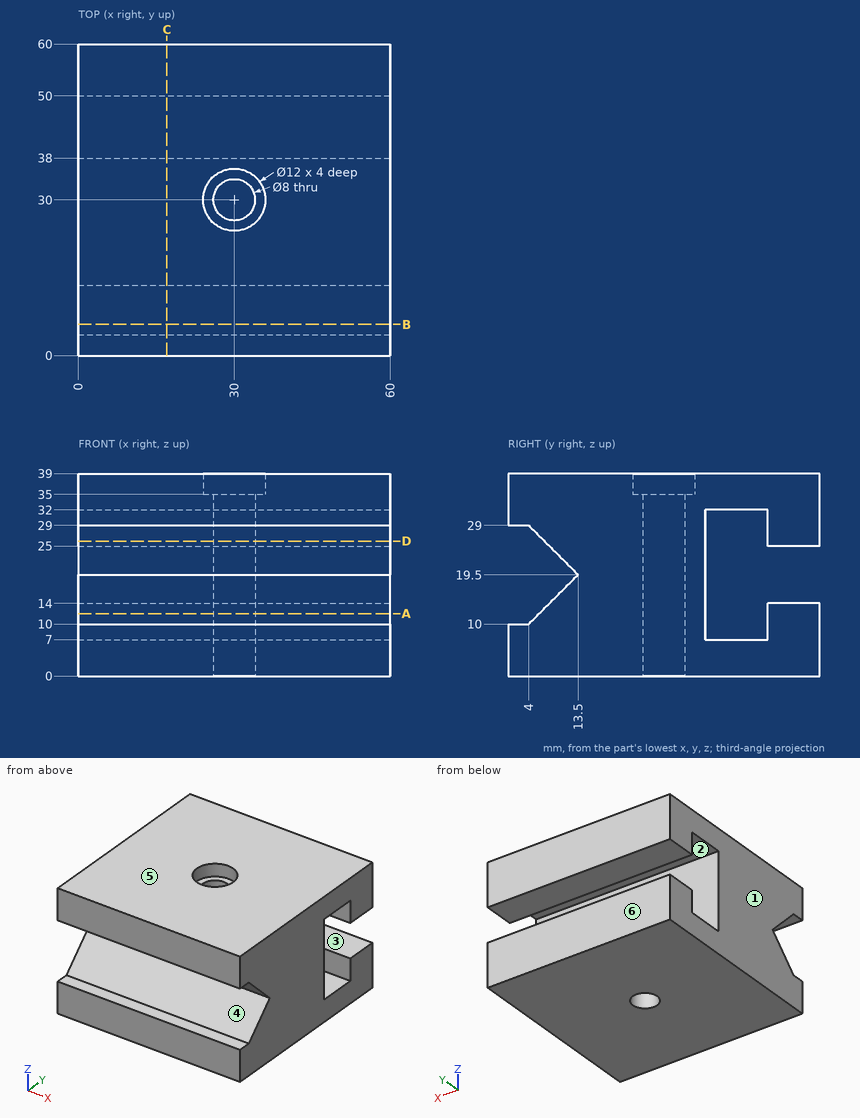
The figure shows three views and two pictorial views of one solid part (mm, origin at its lowest corner). Answer the questions. A direction names the side the tool comes from. Give positions to 0.01 mm unless a question says otherwise; leave off trailing zeros. Loops run counter-clockwise (first coordinate to the right, second up) from the corner with the lowest first, then second, coordinate; pieces in that order, holes last. Notation, with made-up numbers: (8.25, -25.5) -> (58.25, -25.5) arc R20 cw to (58.25, -21.5) -> close; hole circle Ø7 at (62.25, 44.5). An arc over 180 degrees is marked (long way). Use a Markdown table: item, result. Add a question column.
1. A flat-ended cylindrical pin translates along its axis: pin 1 Ø3.5 at (x, y) = (32.5, 27.5) entering from +Z. Find the tip coordinate at first contact, or state that the pin passes through.
2. Determine the mould class of the marked faces 4, 5 and 6 for opening direction Z: released by +Z, released by -Z, zero draft, split by the parting line, or undercut.
3. Find the intervals of material crossed by probe 1 along X at (y, z) = (30, 19); probe 2 along X at (y, z) = (30, 37.6); probe 3 along Z at (x, y) = (17, 55.5), in increasing order.
4. Section D-D on z = 26 is taken. Determine the outline of the cut face in (x, y).
5. For the marked faces 1, 2 and 3, determine the directions among +Z, -Z, +X, -X, +Y, -Y from which every point of the face is accessible in a straight line to the end or side of a thin tool.
6. Section C-C on x = 17 is taken. Determine the outline of the cut face in (y, z), and give its area (3 significant figures).
7. Section B-B on y = 6 is taken. Determine the outline of the cut face in (x, z).
8. Section A-A on z = 12 is taken. Determine the outline of the cut face in (x, y), and give its area (3 significant figures).
Results below:
| question | item | result |
|---|---|---|
| 1 | pin 1 | stops at z = 35 |
| 2 | face 4 | undercut |
| 2 | face 5 | released by +Z |
| 2 | face 6 | zero draft |
| 3 | probe 1 | x = 0 to 26, 34 to 60 |
| 3 | probe 2 | x = 0 to 24, 36 to 60 |
| 3 | probe 3 | z = 0 to 14, 25 to 39 |
| 4 | outline | (0, 7) -> (60, 7) -> (60, 38) -> (0, 38) -> close; (0, 50) -> (60, 50) -> (60, 60) -> (0, 60) -> close; hole circle Ø8 at (30, 30) |
| 5 | face 1 | +Z, -Z, -X, +Y, -Y |
| 5 | face 2 | +X, -X |
| 5 | face 3 | +X, -X, +Y |
| 6 | outline | (0, 0) -> (60, 0) -> (60, 14) -> (50, 14) -> (50, 7) -> (38, 7) -> (38, 32) -> (50, 32) -> (50, 25) -> (60, 25) -> (60, 39) -> (0, 39) -> (0, 29) -> (4, 29) -> (13.5, 19.5) -> (4, 10) -> (0, 10) -> close |
| 6 | area | 1,760 mm^2 |
| 7 | outline | (0, 0) -> (60, 0) -> (60, 12) -> (0, 12) -> close; (0, 27) -> (60, 27) -> (60, 39) -> (0, 39) -> close |
| 8 | outline | (0, 6) -> (60, 6) -> (60, 38) -> (0, 38) -> close; (0, 50) -> (60, 50) -> (60, 60) -> (0, 60) -> close; hole circle Ø8 at (30, 30) |
| 8 | area | 2,470 mm^2 |
